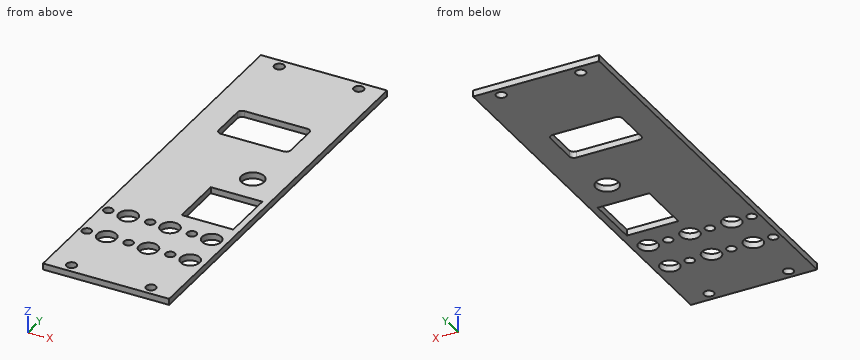
from build123d import *

# Parameters (mm, degrees)
SKETCH2_W           = 40.3
SKETCH2_H           = 128.5
SKETCH2_R           = 1.6
SKETCH2_R_2         = 3.05
SKETCH2_R_3         = 1.5
SKETCH2_R_4         = 3.6
SKETCH2_W_2         = 16.5
SKETCH2_H_2         = 17.2
BOSS_EXTRUDE2_DEPTH = 2


with BuildPart() as part:
    # Sketch2 → Boss-Extrude2 (new body)
    with BuildSketch(Plane.XY):
        with Locations((20.15, 64.25)):
            Rectangle(SKETCH2_W, SKETCH2_H)
        with Locations((7.5, 125.5)):
            Circle(SKETCH2_R, mode=Mode.SUBTRACT)
        with Locations((32.9, 125.5)):
            Circle(SKETCH2_R, mode=Mode.SUBTRACT)
        with Locations((7.5, 3)):
            Circle(SKETCH2_R, mode=Mode.SUBTRACT)
        with Locations((32.9, 3)):
            Circle(SKETCH2_R, mode=Mode.SUBTRACT)
        with Locations((8.79, 34.05)):
            Circle(SKETCH2_R_2, mode=Mode.SUBTRACT)
        with Locations((8.79, 21.35)):
            Circle(SKETCH2_R_2, mode=Mode.SUBTRACT)
        with Locations((22.13, 34.05)):
            Circle(SKETCH2_R_2, mode=Mode.SUBTRACT)
        with Locations((22.13, 21.35)):
            Circle(SKETCH2_R_2, mode=Mode.SUBTRACT)
        with Locations((35.47, 21.35)):
            Circle(SKETCH2_R_2, mode=Mode.SUBTRACT)
        with Locations((35.47, 34.05)):
            Circle(SKETCH2_R_2, mode=Mode.SUBTRACT)
        with Locations((2.44, 34.05)):
            Circle(SKETCH2_R_3, mode=Mode.SUBTRACT)
        with Locations((15.78, 34.05)):
            Circle(SKETCH2_R_3, mode=Mode.SUBTRACT)
        with Locations((29.12, 34.05)):
            Circle(SKETCH2_R_3, mode=Mode.SUBTRACT)
        with Locations((2.44, 21.35)):
            Circle(SKETCH2_R_3, mode=Mode.SUBTRACT)
        with Locations((15.78, 21.35)):
            Circle(SKETCH2_R_3, mode=Mode.SUBTRACT)
        with Locations((29.12, 21.35)):
            Circle(SKETCH2_R_3, mode=Mode.SUBTRACT)
        with Locations((29.99, 68.34)):
            Circle(SKETCH2_R_4, mode=Mode.SUBTRACT)
        with Locations((29.99, 50.22)):
            Rectangle(SKETCH2_W_2, SKETCH2_H_2, mode=Mode.SUBTRACT)
        with BuildLine():
            Line((10.47, 99.59), (30.47, 99.59))
            ThreePointArc((30.47, 99.59), (31.530660172, 99.150660172), (31.97, 98.09))
            Line((31.97, 98.09), (31.97, 87.09))
            ThreePointArc((31.97, 87.09), (31.530660172, 86.029339828), (30.47, 85.59))
            Line((30.47, 85.59), (10.47, 85.59))
            ThreePointArc((10.47, 85.59), (9.409339828, 86.029339828), (8.97, 87.09))
            Line((8.97, 87.09), (8.97, 98.09))
            ThreePointArc((8.97, 98.09), (9.409339828, 99.150660172), (10.47, 99.59))
        make_face(mode=Mode.SUBTRACT)
    extrude(amount=BOSS_EXTRUDE2_DEPTH)


solid = part.part
CAD build for the part. Positions are in the model's coordinates, mm. Give positions to 0.01 mm unless a question says otherwise; leave off trailing zeros. Write each loop counter-clockwise with the first axis right and the second up, starting at its lowest first coordinate (ties: lowest second). Pieces come first, ordered by that corner, then holes. Notation, with made-up numbers: (53, 21) -> (90, 21) arc R16 ccw to (90, 36) -> close; hole circle Ø7 at (65, 4.5). An arc over 180 degrees is marked (long way). Return JSON: item names as keys, results as strings.
Item 1: Band-saw the part on C-C (x = 15.78). List the corners of the cut face in (y, z).
Answer below:
{"outline": "(0, 0) -> (19.85, 0) -> (19.85, 2) -> (0, 2) -> close; (22.85, 0) -> (32.55, 0) -> (32.55, 2) -> (22.85, 2) -> close; (35.55, 0) -> (85.59, 0) -> (85.59, 2) -> (35.55, 2) -> close; (99.59, 0) -> (128.5, 0) -> (128.5, 2) -> (99.59, 2) -> close"}
Item 2: Band-saw the part on B-B (z = 0.4). Give the number of separate pieces and of enclosed holes in the cut face, then the cut area to 3 significant figures.
Answer below:
{"separate pieces": "1", "enclosed holes": "19", "area": "4,280 mm2"}
Item 3: Drill centre lines: probe 1 along Y at (x, z) = (15.78, 1.55); probe 2 along X at (y, z) = (46, 1.65); probe 3 along Y at (x, z) = (29.12, 0.9). Where is each one in solid material? Low to high.
Answer below:
{"probe 1": "y = 0 to 19.85, 22.85 to 32.55, 35.55 to 85.59, 99.59 to 128.5", "probe 2": "x = 0 to 21.74, 38.24 to 40.3", "probe 3": "y = 0 to 19.85, 22.85 to 32.55, 35.55 to 41.62, 58.82 to 64.85, 71.83 to 85.59, 99.59 to 128.5"}
Item 4: Drop flat-ended pins along their axis: pin 1 (0.6 mm diameter, centred on x = 28, z = 1, fed in from -Y); pin 2 (2.5 mm diameter, centred on x = 15.78, y = 21.35, fed in from -Z). Give the stop position or say it passes through.
Answer below:
{"pin 1": "stops at y = 0", "pin 2": "passes through"}
Item 5: Band-saw the part on D-D (y = 3). List the corners of the cut face in (x, z).
Answer below:
{"outline": "(0, 0) -> (5.9, 0) -> (5.9, 2) -> (0, 2) -> close; (9.1, 0) -> (31.3, 0) -> (31.3, 2) -> (9.1, 2) -> close; (34.5, 0) -> (40.3, 0) -> (40.3, 2) -> (34.5, 2) -> close"}
Item 6: Band-saw the part on A-A (y = 90). List the corners of the cut face in (x, z), then the cut area to 3 significant figures.
Answer below:
{"outline": "(0, 0) -> (8.97, 0) -> (8.97, 2) -> (0, 2) -> close; (31.97, 0) -> (40.3, 0) -> (40.3, 2) -> (31.97, 2) -> close", "area": "34.6 mm2"}
